Geometry: see drawing. Coordinates: mm, zero at the bounding-box minimum. Give positions to 0.01 mm unless a question says otherwise; leave off trailing zeros. Order: outer loops, then holes, each group sorted by start corner. A loop starts at its lowest first (then second) coordinate and runs counter-clockwise, first axis right, second up. Notation, with made-up numbers: (79.25, -16.5) - (85.25, -16.5) arc R8 cw to (85.25, -8.5) - close; hole circle Ø4 at (31, -10.75). An arc over 180 degrees is marked (long way). Write each question's results on one line, items separated by ' | '. Start each with the question number.
Item 1: Section A-A on z = 16. Output: boundary loops of the cut face in (x, y), and give its area (3 significant figures).
Item 2: Line query: line 1 along Y through (x, z) = (21.5, 26.5); line 2 along Z through (x, y) = (5, 20.4); line 3 along Y through (x, z) = (14, 15.5). Output: solid intervals per line, ascending.
Item 3: Section C-C on y = 9. Output: boundary loops of the cut face in (x, z).
Item 4: Section D-D on x = 27. Output: boundary loops of the cut face in (y, z), and give its area (3 significant figures).
Item 5: Contact query for flat-ended pins moving along their axis: pin 1 Ø4 at (x, z) = (12.5, 26) entering from -Y; pin 2 Ø1.6 at (x, z) = (27, 16.5) entering from +Y; pin 3 Ø1 at (x, z) = (5, 16) entering from +Y. Output: stop coordinate, or through.
Item 6: Section B-B on x = 16. Output: boundary loops of the cut face in (y, z).
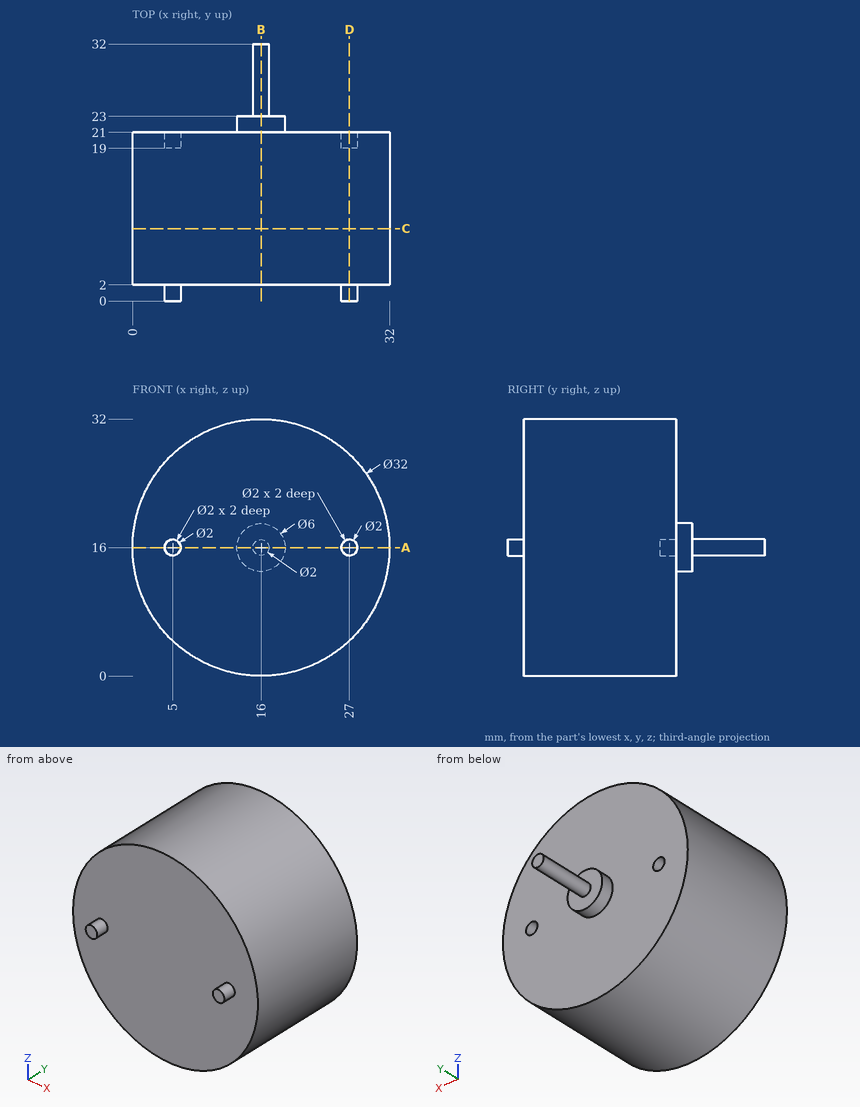
Evaluation:
1) outline: (0, 2) - (4, 2) - (4, 0) - (6, 0) - (6, 2) - (26, 2) - (26, 0) - (28, 0) - (28, 2) - (32, 2) - (32, 21) - (28, 21) - (28, 19) - (26, 19) - (26, 21) - (19, 21) - (19, 23) - (17, 23) - (17, 32) - (15, 32) - (15, 23) - (13, 23) - (13, 21) - (6, 21) - (6, 19) - (4, 19) - (4, 21) - (0, 21) - close | area: 638 mm^2
2) line 1: y = 2 to 21 | line 2: z = 4.38 to 15, 17 to 27.62 | line 3: y = 2 to 23
3) outline: circle Ø32 at (16, 16)
4) outline: (0, 15) - (2, 15) - (2, 4.38) - (21, 4.38) - (21, 15) - (19, 15) - (19, 17) - (21, 17) - (21, 27.62) - (2, 27.62) - (2, 17) - (0, 17) - close | area: 442 mm^2
5) pin 1: stops at y = 2 | pin 2: stops at y = 21 | pin 3: stops at y = 19
6) outline: (2, 0) - (21, 0) - (21, 13) - (23, 13) - (23, 15) - (32, 15) - (32, 17) - (23, 17) - (23, 19) - (21, 19) - (21, 32) - (2, 32) - close
